CAD build for the part. Positions are in the model's coordinates, mm. Coordinates: 2 decimals unless noted, no trailing zeros. Put each result on its own line as item: value. Start each with the question number.
```python
from build123d import *

# Parameters (mm, degrees)
F1_DEPTH = 25.4
F2_R     = 5.08
F3_R     = 5.08


with BuildPart() as f1:
    # F0 (on Front) → F1 (new body)
    with BuildSketch(Plane.XZ):
        Polygon((118.762286, 37.117315), (-135.237714, 37.117315), (-135.237714, -64.482685), (118.762286, -64.877713), align=None)
    extrude(amount=F1_DEPTH)

    # F2
    f2_edges = [f1.edges().sort_by_distance(p)[0] for p in [
        (-135.237714, -12.7, 37.117315),
    ]]
    fillet(f2_edges, radius=F2_R)

    # F3
    f3_edges = [f1.edges().sort_by_distance(p)[0] for p in [
        (118.762286, -12.7, 37.117315),
        (118.762286, -12.7, -64.877713),
        (-135.237714, -12.7, -64.482685),
    ]]
    fillet(f3_edges, radius=F3_R)


solid = f1.part
```
(1) Drop flat-ended pins along their axis: pin 1 (4 mm diameter, centred on x = -42, z = -6.5, fed in from +Y); pin 2 (5 mm diameter, centred on x = -100.5, y = -6, fed in from -Z). Give the stop position or say it passes through.
(2) Drill centre lines: line 1 (Z direction, x = -124.5, y = -4.5); line 2 (Z direction, x = 97.5, y = -1.5). Where is each one in solid material? Low to high. Write a range as [from, to].
(3) Two-plate mould, pull along X, no slides. Class faces 1 (the face through (-135.238, -13, -13)), 2 (the face through (118.762, -13, -15)), 3 (the face through (-10, 0, -13)): +X half, -X half, draft (parallel to the pull), parting line (faces both ways), or undercut.
Result set:
1. pin 1: stops at y = 0
1. pin 2: stops at z = -64.54
2. line 1: z = [-64.5, 37.12]
2. line 2: z = [-64.84, 37.12]
3. face 1: -X half
3. face 2: +X half
3. face 3: draft
